Check sheet for the modelled part. Datum: model origin and axes. Units: mm. A direction names the side the tool comes from. Round coordinates to 2 decimals unless told otherwise and drop trailing zeros. Order: outer loops, then holes, each group sorted by start corner. A loop starts at its lowest first (then second) coordinate and runs counter-clockwise, first axis right, second up. Notation, with made-up numbers: M -4.5,27.5 L 7.5,27.5 A21 cw 7.5,57.5 Z; hole C 34.25,16 d5. An arc over 180 degrees is marked long. One line per item, written item: value. Start each with the question number.
(1) Cross-section at D-D, the plane y = -11. Enter the section's corners in (x, z), and give its area (3 significant figures).
(2) Thickness scan on L1, parallel to Y at x = -24, z = 3.75; L2, parallel to X at y = 13, z = 1.1; L3, parallel to X at y = 1, z = 1. Record the ranges inside material, lowest first.
(3) Depth check by flat-ended pin: pin 1 Ø2 at (x, z) = (25.5, 4.5) entering from +Y; pin 2 Ø1.5 at (x, z) = (20, 1.5) entering from -Y; pin 3 Ø3.5 at (x, y) = (30.12, 0) entering from -Z; pin 4 Ø3 at (y, z) = (-12, 4.5) entering from +X. Enter the tip coordinate at first touch or a pass-through.
(4) Release check for a two-part mould opening along Y. For faces 4 (the face through (0, 15, 2)), 5 (the face through (28.12, 0.09, 2.46)), 6 (the face through (8, -12, 2)) record: released by +Y, released by -Y, zero draft, split by the parting line, or undercut.
(5) Cross-section at C-C, the plane x = -25. Enter the section's corners in (y, z).
(6) Cross-section at A-A, the plane z = 0.9. Enter the section's corners in (x, y).
(7) Access from +Z, -Z, +X, -X, +Y, -Y to the whole of each face (thin tool, end or side, straight path). Record for faces 1 (the face through (-8, 12, 2)), 2 (the face through (-8, -13, 2)), 3 (the face through (8, 13, 2)).
(8) Cross-section at B-B, the plane y = 0. Enter the section's corners in (x, z), and give its area (3 significant figures).
from build123d import *

# Parameters (mm, degrees)
SKETCH1_R           = 2
BOSS_EXTRUDE1_DEPTH = 5


with BuildPart() as part:
    # Sketch1 → Boss-Extrude1 (new body)
    with BuildSketch(Plane.XY):
        Polygon((-8, 10), (-8, 15), (8, 15), (8, 10), (38, 10), (38, -10), (8, -10), (8, -15), (-8, -15), (-8, -10), (-38, -10), (-38, 10), align=None)
        with Locations((30.117717463, 0)):
            Circle(SKETCH1_R, mode=Mode.SUBTRACT)
    extrude(amount=BOSS_EXTRUDE1_DEPTH)


solid = part.part
Values found:
1. outline: M -8,0 L 8,0 L 8,5 L -8,5 Z
1. area: 80.0 mm^2
2. L1: -10 to 10
2. L2: -8 to 8
2. L3: -38 to 28.39, 31.85 to 38
3. pin 1: y = 10
3. pin 2: y = -10
3. pin 3: through
3. pin 4: x = 8
4. face 4: released by +Y
4. face 5: undercut
4. face 6: zero draft
5. outline: M -10,0 L 10,0 L 10,5 L -10,5 Z
6. outline: M -38,-10 L -8,-10 L -8,-15 L 8,-15 L 8,-10 L 38,-10 L 38,10 L 8,10 L 8,15 L -8,15 L -8,10 L -38,10 Z; hole C 30.12,0 d4
7. face 1: +Z, -Z, -X, +Y
7. face 2: +Z, -Z, -X, -Y
7. face 3: +Z, -Z, +X, +Y
8. outline: M -38,0 L 28.12,0 L 28.12,5 L -38,5 Z; M 32.12,0 L 38,0 L 38,5 L 32.12,5 Z
8. area: 360 mm^2
